```python
from build123d import *

# Parameters (mm, degrees)
SKETCH1_W           = 95.89
SKETCH1_H           = 90.17
SUBSTRATE_DEPTH     = 1.6
SKETCH2_R           = 1.5
CUT_EXTRUDE2_DEPTH  = 10
SKETCH3_W           = 1.2
SKETCH3_H           = 1.2
SKETCH3_W_2         = 1
SKETCH3_H_2         = 1
BOSS_EXTRUDE1_DEPTH = 10
SKETCH4_OUTSIDE_W   = 124.318
SKETCH4_OUTSIDE_H   = 118.598
CUT_EXTRUDE3_DEPTH  = 10
SKETCH5_R           = 1.5
CUT_EXTRUDE4_DEPTH  = 10


with BuildPart() as part:
    # Sketch1 → Substrate (new body)
    with BuildSketch(Plane(origin=(0, 0, 0), x_dir=(1, 0, 0), z_dir=(0, 1, 0))):
        Rectangle(SKETCH1_W, SKETCH1_H)
    extrude(amount=SUBSTRATE_DEPTH)

    # Sketch2 → Cut-Extrude2 (cut)
    with BuildSketch(Plane(origin=(0, 1.6, 0), x_dir=(1, 0, 0), z_dir=(0, 1, 0))):
        with Locations(Location((42.845, 36.085, 0), (0, 0, 270))):
            Circle(SKETCH2_R)
        with Locations(Location((42.845, -37.585, 0), (0, 0, 270))):
            Circle(SKETCH2_R)
        with Locations(Location((-42.945, -39.985, 0), (0, 0, 270))):
            Circle(SKETCH2_R)
        with Locations(Location((-42.945, 39.985, 0), (0, 0, 270))):
            Circle(SKETCH2_R)
    extrude(amount=-CUT_EXTRUDE2_DEPTH, mode=Mode.SUBTRACT)

    # Sketch3 → Boss-Extrude1 (add)
    with BuildSketch(Plane(origin=(0, 1.6, 0), x_dir=(1, 0, 0), z_dir=(0, 1, 0))):
        Rectangle(SKETCH3_W, SKETCH3_H)
        Rectangle(SKETCH3_W_2, SKETCH3_H_2, mode=Mode.SUBTRACT)
    extrude(amount=BOSS_EXTRUDE1_DEPTH)

    # Sketch4 outside → Cut-Extrude3 (cut)
    with BuildSketch(Plane(origin=(0, 1.6, 0), x_dir=(1, 0, 0), z_dir=(0, 1, 0))):
        Rectangle(SKETCH4_OUTSIDE_W, SKETCH4_OUTSIDE_H)
        with BuildLine():
            Line((-42.677096043, -44.977817588), (42.845, -42.685))
            ThreePointArc((42.845, -42.685), (46.451244584, -41.191244584), (47.945, -37.585))
            Line((47.945, -37.585), (47.945, 36.085))
            ThreePointArc((47.945, 36.085), (46.451244584, 39.691244584), (42.845, 41.185))
            Line((42.845, 41.185), (-42.502925272, 44.965418651))
            ThreePointArc((-42.502925272, 44.965418651), (-46.320620414, 43.673520953), (-47.945, 39.985))
            Line((-47.945, 39.985), (-47.945, -39.985))
            ThreePointArc((-47.945, -39.985), (-46.384511609, -43.614016381), (-42.677096043, -44.977817588))
        make_face(mode=Mode.SUBTRACT)
    extrude(amount=-CUT_EXTRUDE3_DEPTH, mode=Mode.SUBTRACT)

    # Sketch5 → Cut-Extrude4 (cut)
    with BuildSketch(Plane(origin=(0, 1.6, 0), x_dir=(1, 0, 0), z_dir=(0, 1, 0))):
        with Locations(Location((-35.1, 35.1, 0), (0, 0, 270))):
            Circle(SKETCH5_R)
        with Locations(Location((35.1, 35.1, 0), (0, 0, 270))):
            Circle(SKETCH5_R)
        with Locations(Location((35.1, -35.1, 0), (0, 0, 270))):
            Circle(SKETCH5_R)
        with Locations(Location((-35.1, -35.1, 0), (0, 0, 270))):
            Circle(SKETCH5_R)
    extrude(amount=-CUT_EXTRUDE4_DEPTH, mode=Mode.SUBTRACT)


solid = part.part
```
For this review, take the finished solid that the model builds, in its own axes (mm). Give positions to 0.01 mm unless a question says otherwise; leave off trailing zeros. Loops run counter-clockwise (first coordinate to the right, second up) from the corner with the lowest first, then second, coordinate; pieces in that order, holes last. Notation, with made-up numbers: M 38.5,1 L 65.5,1 A25 ccw 65.5,31 Z; hole C 13.25,30.5 d7. An arc over 180 degrees is marked long. One line per item, written item: value. Start each with the question number.
Q1. For L1, parallel to X at y = 1, z = 35.1 (3 decimals); L2, parallel to Z at x = -42.5, y = 1; L3, parallel to Y at x = -8.5, z = -19.5, list the stretches that pass through material, from the lowest coordinate up.
Q2. Clearance check with flat-ended pins moving along their axes: pin 1 Ø12 at (x, z) = (37.5, -30) entering from +Y; pin 2 Ø6 at (x, y) = (-35, 2.5) entering from +Z; pin 3 Ø0.6 at (x, y) = (0, 5) entering from -Z. State where each tip first meets the part, or that it passes through.
Q3. Draft analysis for pull direction X (two halves, no side actions). For faces 1 (the face through (43.86, 0.81, 36.48)), 2 (the face through (46.41, 0.81, 41.23)), 3 (the face through (-1, 0, -1)), state which applies: released by +X, released by -X, zero draft, split by the parting line, or undercut.
Q4. Add section C-C (x = 35.1). Give the boundary of the cut face in (y, z).
Q5. Add section B-B (x = -35.1). Give the boundary of the cut face in (y, z), and give its area (3 significant figures).
Q6. Add section D-D (z = 14). Give the boundary of the cut face in (x, y) (3 decimals).
Q7. Add section A-A (y = 4). Give the boundary of the cut face in (x, z), and give its area (3 significant figures).
Reply:
1. L1: -47.945 to -36.6, -33.6 to 33.6, 36.6 to 47.945
1. L2: -44.97 to -41.42, -38.55 to 38.55, 41.42 to 44.97
1. L3: 0 to 1.6
2. pin 1: y = 1.6
2. pin 2: z = 44.85
2. pin 3: z = -0.6
3. face 1: undercut
3. face 2: released by +X
3. face 3: zero draft
4. outline: M 0,-41.53 L 1.6,-41.53 L 1.6,-36.6 L 0,-36.6 Z; M 0,-33.6 L 1.6,-33.6 L 1.6,33.6 L 0,33.6 Z; M 0,36.6 L 1.6,36.6 L 1.6,42.89 L 0,42.89 Z
5. outline: M 0,-44.64 L 1.6,-44.64 L 1.6,-36.6 L 0,-36.6 Z; M 0,-33.6 L 1.6,-33.6 L 1.6,33.6 L 0,33.6 Z; M 0,36.6 L 1.6,36.6 L 1.6,44.77 L 0,44.77 Z
5. area: 133 mm²
6. outline: M -47.945,0 L 47.945,0 L 47.945,1.6 L -47.945,1.6 Z
7. outline: M -0.6,-0.6 L 0.6,-0.6 L 0.6,0.6 L -0.6,0.6 Z; hole M -0.5,-0.5 L 0.5,-0.5 L 0.5,0.5 L -0.5,0.5 Z
7. area: 0.440 mm²
